from build123d import *

# Parameters (mm, degrees)
BOSS_EXTRUDE1_DEPTH = 2
SKETCH2_R           = 2
BOSS_EXTRUDE2_DEPTH = 8
SKETCH5_R           = 2
CUT_EXTRUDE2_DEPTH  = 4


with BuildPart() as part:
    # Sketch1 → Boss-Extrude1 (new body)
    with BuildSketch(Plane.XY):
        with BuildLine():
            Line((0, -2.5), (34, -2.5))
            ThreePointArc((34, -2.5), (36.5, 0), (34, 2.5))
            Line((34, 2.5), (0, 2.5))
            ThreePointArc((0, 2.5), (-2.5, 0), (0, -2.5))
        make_face()
    extrude(amount=BOSS_EXTRUDE1_DEPTH)

    # Sketch2 → Boss-Extrude2 (add)
    with BuildSketch(Plane.XY.offset(2)):
        Circle(SKETCH2_R)
    extrude(amount=BOSS_EXTRUDE2_DEPTH)

    # Sketch5 → Cut-Extrude2 (cut, symmetric)
    with BuildSketch(Plane(origin=(0, 0, 0), x_dir=(-1, 0, 0), z_dir=(0, 0, -1))):
        with Locations(Location((-34, 0, 0), (0, 0, 180))):
            Circle(SKETCH5_R)
    extrude(amount=CUT_EXTRUDE2_DEPTH, both=True, mode=Mode.SUBTRACT)


solid = part.part
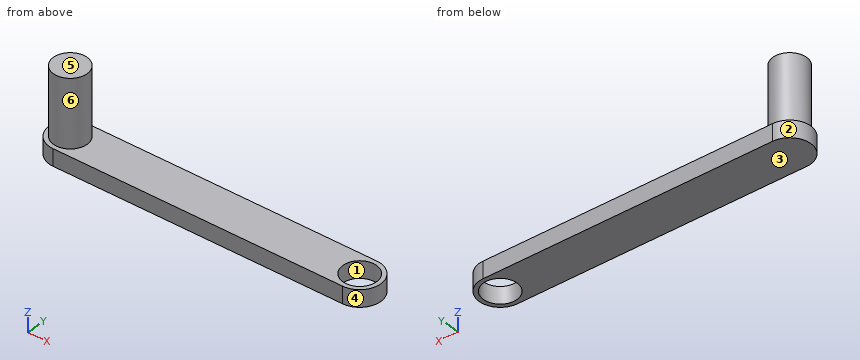
The model under review builds one solid part; all positions refer to its coordinate system, in mm. Face numbers are marked on the shaded views. A direction names the side the tool comes from. Round coordinates to 2 decimals unless told otherwise and drop trailing zeros. Write each loop counter-clockwise with the first axis right and the second up, starting at its lowest first coordinate (ties: lowest second). Pieces come first, ordered by that corner, then holes. Notation, with made-up numbers: M 26.25,16 L 48.25,16 A29 cw 48.25,37 Z; hole C -4,19.25 d10. An arc over 180 degrees is marked long. Use a Markdown table: item, result. Add a question column.
Q1. We need section C-C, the plane x = 31. State the section outline as (y, z) points.
Q2. The part is to be moulded in two halves that separate along X. For the marked faces 1, 2, 3 and 4, say which applies: pulls with the +X half, pulls with the -X half, needs draft (parallel to the pull), parting line crosses it, or undercut.
Q3. Machinability: for the marked faces 5 and 6, which of the approach directions +Z, -Z, +X, -X, +Y, -Y give a long, thin tool a straight path to every point of the face, cutting with its end or side? Answer none if there is none.
Q4. We need section B-B, the plane z = 5.75. State the section outline as (x, y) points.
Q5. We need section A-A, the plane y = 0. State the section outline as (x, z) points, plus the area to 3 significant figures.
Q6. To check wall thickness, follow line 1 (Y direction, x = 34, z = 0.65); line 2 (Z direction, x = 17.5, y = -0.35); line 3 (X direction, y = -0.6, z = 1.5). State the ranges of each line that lie inside material, in increasing order.
Q7. Insertion check: pin 1 (2.5 mm diameter, centred on x = 22.5, y = 0, fed in from +Z). The pin has a flat end and moves straight along its axis. Give the tip position at first contact, or say it passes through.
Findings below:
| question | item | result |
|---|---|---|
| 1 | outline | M -2.5,0 L 2.5,0 L 2.5,2 L -2.5,2 Z |
| 2 | face 1 | undercut |
| 2 | face 2 | pulls with the -X half |
| 2 | face 3 | needs draft |
| 2 | face 4 | pulls with the +X half |
| 3 | face 5 | +Z, +X, -X, +Y, -Y |
| 3 | face 6 | +Z |
| 4 | outline | C 0,0 d4 |
| 5 | outline | M -2.5,0 L 32,0 L 32,2 L 2,2 L 2,10 L -2,10 L -2,2 L -2.5,2 Z; M 36,0 L 36.5,0 L 36.5,2 L 36,2 Z |
| 5 | area | 102 mm² |
| 6 | line 1 | y = -2.5 to -2, 2 to 2.5 |
| 6 | line 2 | z = 0 to 2 |
| 6 | line 3 | x = -2.43 to 32.09, 35.91 to 36.43 |
| 7 | pin 1 | stops at z = 2 |
